from build123d import *

# Parameters (mm, degrees)
F0_R     = 19.05
F1_DEPTH = 9.525
F2_SIZE2 = 3.6661742094
F2_SIZE  = 6.35
F3_SIZE2 = 3.6661742094
F3_SIZE  = 6.35


# Not quite as in the source:
# - a length typed as a fraction of an inch, garbled in the dataset ("3 / 203.2 mm" for 3/8 in), is restored


with BuildPart() as f1:
    # F0 (on Front) → F1 (new body)
    with BuildSketch(Plane.XZ):
        Polygon((68.2071738782, 117.0869429827), (-84.1928261218, 117.0869429827), (-84.1928261218, -86.1130570173), (119.0071738782, -86.1130570173), (119.0071738782, 66.2869429827), align=None)
        Polygon((14.2321738782, -54.3630570173), (42.8071738782, -3.5630570173), (71.3821738782, -54.3630570173), align=None, mode=Mode.SUBTRACT)
        with Locations((47.5696738782, 53.5869429827)):
            Circle(F0_R, mode=Mode.SUBTRACT)
    extrude(amount=F1_DEPTH)

    # F2
    f2_edges = [f1.edges().sort_by_distance(p)[0] for p in [
        (119.007174, -9.525, -9.913057),
    ]]
    f2_side = f1.faces().sort_by_distance((119.007174, -4.7625, -9.913057))[0]
    chamfer(f2_edges, length=F2_SIZE, length2=F2_SIZE2, reference=f2_side)

    # F3
    f3_edges = [f1.edges().sort_by_distance(p)[0] for p in [
        (-84.192826, -9.525, 15.486943),
    ]]
    f3_side = f1.faces().sort_by_distance((-84.192826, -4.7625, 15.486943))[0]
    chamfer(f3_edges, length=F3_SIZE, length2=F3_SIZE2, reference=f3_side)


solid = f1.part
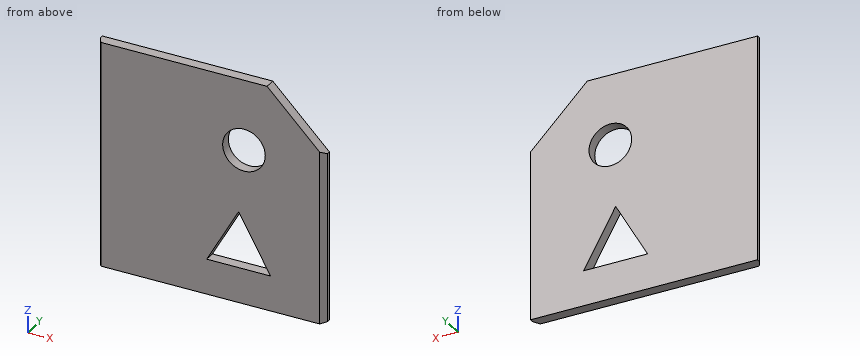
Could you check a few things on this model? Use its own coordinates, in mm. Give positions to 0.01 mm unless a question says otherwise; leave off trailing zeros. Order: outer loops, then holes, each group sorted by start corner. A loop starts at its lowest first (then second) coordinate and runs counter-clockwise, first axis right, second up. Notation, with made-up numbers: M -24.75,-6 L 23.25,-6 A36 cw 23.25,28 Z; hole C 64,-28 d4. An arc over 180 degrees is marked long. One line per question, with ' | ' between items.
1. I'm going to push flat-ended pins straight in: pin 1 (2 mm diameter, centred on y = -7.5, z = -40.5, fed in from -X); pin 2 (4 mm diameter, centred on x = 13, z = 20.5, fed in from +Y); pin 3 (5 mm diameter, centred on y = -6, z = 25.5, fed in from -X). Where does each tip first touch, or does it pass through?
Results:
pin 1: x = -82.27 | pin 2: y = 0 | pin 3: x = -84.01
2. I want a section at C-C (y = -5.5). List the corners of the cut face in (x, z) for me.
Results:
outline: M -82.85,-86.11 L 117.66,-86.11 L 117.66,67.63 L 68.21,117.09 L -82.85,117.09 Z; hole M 14.23,-54.36 L 71.38,-54.36 L 42.81,-3.56 Z; hole C 47.57,53.59 d38.1
3. I want a section at B-B (x = 48). List the corners of the cut face in (y, z) for me (3 decimals), and give its area (3 significant figures).
Results:
outline: M -9.525,-86.113 L 0,-86.113 L 0,-54.363 L -9.525,-54.363 Z; M -9.525,-12.795 L 0,-12.795 L 0,34.542 L -9.525,34.542 Z; M -9.525,72.632 L 0,72.632 L 0,117.087 L -9.525,117.087 Z | area: 1,180 mm²
4. If I drill on line 1 (Z direction, x = 50.5, y = -6.25); line 2 (Z direction, x = 45, y = -7.25); line 3 (X direction, y = -4.75, z = -19.5), over which ranges is the centre line in solid material (lowest first)?
Results:
line 1: -86.11 to -54.36, -17.24 to 34.76, 72.41 to 117.09 | line 2: -86.11 to -54.36, -7.46 to 34.71, 72.46 to 117.09 | line 3: -83.28 to 33.84, 51.77 to 118.1
5. I want a section at D-D (z = 61). List the corners of the cut face in (x, y) for me (3 decimals).
Results:
outline: M -84.193,-3.175 L -80.527,-9.525 L 30.021,-9.525 L 30.021,0 L -84.193,0 Z; M 65.118,-9.525 L 115.341,-9.525 L 119.007,-3.175 L 119.007,0 L 65.118,0 Z
6. I want a section at A-A (z = -43). List the corners of the cut face in (x, y) for me (3 decimals), and give its area (3 significant figures).
Results:
outline: M -84.193,-3.175 L -80.527,-9.525 L 20.624,-9.525 L 20.624,0 L -84.193,0 Z; M 64.99,-9.525 L 115.341,-9.525 L 119.007,-3.175 L 119.007,0 L 64.99,0 Z | area: 1,490 mm²
